CAD build for the part. Positions are in the model's coordinates, mm. A direction names the side the tool comes from. Coordinates: 2 decimals unless noted, no trailing zeros. Loops run counter-clockwise (first coordinate to the right, second up) from the corner with the lowest first, then second, coordinate; pieces in that order, holes last. Notation, with made-up numbers: (28.5, 71) -> (57.5, 71) arc R14 ccw to (57.5, 80) -> close; hole circle Ø11 at (15.25, -1.75). An arc over 180 degrees is marked (long way). Answer as a JSON object with one key per item and string values. Group by question number.
Solid Edge part; units mm, degrees
sketch "Sketch1" plane through (0, 0, 0) normal (0, 0, 1) x (1, 0, 0)
  circle A0 centre (0, 0) radius 5
extrude "Protrusion1" add sketch "Sketch1" along normal blind 25
sketch "Sketch2" plane through (0, 0.5, 25) normal (0, 0, 1) x (1, 0, 0)
  circle A0 centre (0, -0.5) radius 5
extrude "ExtrudedProtrusion_2" add sketch "Sketch2" along normal blind 110
sketch "Sketch3" plane through (0, 0, 135) normal (0, 0, 1) x (0, 1, 0)
  line L0 (4, 1.5) -> (6, 1.5)
  line L1 (6, 1.5) -> (6, -1.5)
  line L2 (6, -1.5) -> (4, -1.5)
  line L3 (4, -1.5) -> (4, 1.5)
  circle A0 centre (0, 0) radius 5
extrude "ExtrudedProtrusion_4" add sketch "Sketch3" along normal blind 32
sketch "Sketch4" plane through (0, 0.5, 167) normal (0, 0, 1) x (-1, 0, 0)
  circle A0 centre (0, 0.5) radius 5
extrude "ExtrudedProtrusion_5" add sketch "Sketch4" along normal blind 10
sketch "Sketch5" plane through (0, 5.3848, 135) normal (0, 0, -1) x (-1, 0, 0)
  circle A0 centre (0, -5.3848) radius 6.2
extrude "ExtrudedProtrusion_6" add sketch "Sketch5" along normal blind 3
properties material "Aluminum, 1060"
Item 1: Band-saw the part on B-B, the plane z = 72.5. List the corners of the cut face in (x, y).
Item 2: Band-saw the part on A-A, the plane x = 0. List the corners of the cut face in (y, z).
Item 3: Flat gauge pins, fed straight in: P1, Ø2.5, axis at x = 0.5, z = 143.5, coming from the +Y side; P2, Ø6, axis at x = 0.5, z = 126, coming from the -Y side; P3, Ø3, axis at y = 4, z = 77, coming from the -X side. Where does each tip first touch, or does it go through?
Item 4: 3-axis set-ups, long thin cutter, end or side, ignore diameter. For faces 1 (the cylindrical face through (-1.08, 4.88, 65.08)), 2 (the flat face through (0, 6, 151)), 3 (the cylindrical face through (-2.86, 5.5, 133.52)), 4 (the flat face through (0, 0, 0)), 5 (the cylindrical face through (-4.995, -0.225, 155.706)): which of +Z, -Z, +X, -X, +Y, -Y reach the whole face in a straight line?
Item 5: Band-saw the part on D-D, the plane z = 162.5. List the corners of the cut face in (x, y), and give its area (3 significant figures).
Item 6: Drill centre lines: L1, parallel to Z at x = -4.5, y = 3.75; L2, parallel to X at y = 3, z = 80; L3, parallel to X at y = -3.5, z = 91. Where is each one in solid material? Low to high.
Item 7: Band-saw the part on C-C, the plane y = -2. List the corners of the cut face in (x, z), and give its area (3 significant figures).
Reply:
{
 "1": {"outline": "circle Ø10 at (0, 0)"},
 "2": {"outline": "(-6.2, 132) -> (-5, 132) -> (-5, 0) -> (5, 0) -> (5, 132) -> (6.2, 132) -> (6.2, 135) -> (6, 135) -> (6, 167) -> (5, 167) -> (5, 177) -> (-5, 177) -> (-5, 135) -> (-6.2, 135) -> close"},
 "3": {"P1": "y = 6", "P2": "y = -5", "P3": "x = -4.33"},
 "4": {"face 1": "-Z", "face 2": "+Z, +X, -X, +Y", "face 3": "+Z, -Z", "face 4": "-Z, +X, -X, +Y, -Y", "face 5": "+Z"},
 "5": {"outline": "(-1.5, 4.77) arc R5 ccw (long way) to (1.5, 4.77) -> (1.5, 6) -> (-1.5, 6) -> close", "area": "81.8 mm²"},
 "6": {"L1": "132 to 135", "L2": "-4 to 4", "L3": "-3.57 to 3.57"},
 "7": {"outline": "(-5.87, 132) -> (-4.58, 132) -> (-4.58, 0) -> (4.58, 0) -> (4.58, 132) -> (5.87, 132) -> (5.87, 135) -> (4.58, 135) -> (4.58, 177) -> (-4.58, 177) -> (-4.58, 135) -> (-5.87, 135) -> close", "area": "1,630 mm²"}
}
